Source: CAD feature listing. Evaluate the final solid. Frame: model axes, mm. Coordinates: 2 decimals unless noted, no trailing zeros. Loops run counter-clockwise (first coordinate to the right, second up) from the corner with the lowest first, then second, coordinate; pieces in that order, holes last. Notation, with made-up numbers: (-32.5, 33) - (18.5, 33) arc R27 cw to (18.5, 57) - close; hole circle Ø1 at (31.25, 40.5). An arc over 180 degrees is marked (long way). Use CSV: the item, a comma, the result in double quotes. Start each with the question number.
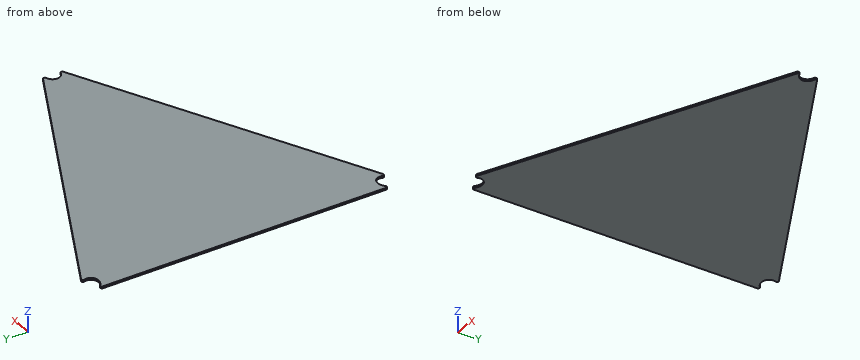
```python
from build123d import *

# Parameters (mm, degrees)
BOSS_EXTRUDE1_DEPTH = 3.175
FILLET1_START       = -1
FILLET1_DEPTH       = 5


with BuildPart() as part:
    # Sketch2 → Boss-Extrude1 (new body)
    with BuildSketch(Plane.XY):
        with BuildLine():
            Line((252.882647522, 18.233509916), (-227.808389099, 261.102259727))
            add(Edge.make_bspline(
                [(-227.808389099, 261.102259727), (-218.508408171, 256.403452033), (-217.090340448, 248.048262702), (-220.367085383, 242.285684549)],
                knots=[0.742781474, 0.742781474, 0.742781474, 0.742781474, 1, 1, 1, 1], degree=3, weights=[0.500416857, 0.490514251, 0.657041966, 1]))
            add(Edge.make_bspline(
                [(-220.367085383, 242.285684549), (-227.805809429, 229.203729887), (-247.735230176, 231.479633917), (-247.728634027, 251.479512649)],
                knots=[0, 0, 0, 0, 0.406744285, 0.406744285, 0.406744285, 0.406744285], degree=3, weights=[1, 0.457674286, 0.356524342, 0.696550168]))
            Line((-247.728634027, 251.479512649), (-247.88971408, -236.923885776))
            add(Edge.make_bspline(
                [(-247.88971408, -236.923885776), (-247.883118871, -216.926855588), (-227.957336221, -214.663599199), (-220.525871765, -227.745847533)],
                knots=[0.593296933, 0.593296933, 0.593296933, 0.593296933, 1, 1, 1, 1], degree=3, weights=[0.696446809, 0.356544847, 0.457729245, 1]))
            add(Edge.make_bspline(
                [(-220.525871765, -227.745847533), (-217.251599097, -233.509832332), (-218.672940969, -241.864237022), (-227.974334939, -246.55870873)],
                knots=[0, 0, 0, 0, 0.25721856, 0.25721856, 0.25721856, 0.25721856], degree=3, weights=[1, 0.65704192, 0.490514207, 0.500416861]))
            Line((-227.974334939, -246.55870873), (252.876255857, -3.870408269))
            add(Edge.make_bspline(
                [(252.876255857, -3.870408269), (240.565044662, -10.083953555), (231.629829811, -2.056184754), (231.628366282, 7.18068181)],
                knots=[0.684200569, 0.684200569, 0.684200569, 0.684200569, 1, 1, 1, 1], degree=3, weights=[0.534636521, 0.423812933, 0.578934092, 1]))
            add(Edge.make_bspline(
                [(231.628366282, 7.18068181), (231.626901898, 16.422942754), (240.567824747, 24.455563967), (252.882647522, 18.233509916)],
                knots=[0, 0, 0, 0, 0.315906176, 0.315906176, 0.315906176, 0.315906176], degree=3, weights=[1, 0.578791765, 0.423708096, 0.534748993]))
        make_face()
    extrude(amount=BOSS_EXTRUDE1_DEPTH)

    # Fillet1: read off the stored shape, not the designer's step
    # Fillet1 outline → Fillet1 (cut)
    with BuildSketch(Plane.XY.offset(FILLET1_START)):
        with BuildLine():
            Line((-247.728634027, 251.479512649), (-247.73250842, 239.732143832))
            ThreePointArc((-247.73250842, 239.732143832), (-246.154410329, 242.082124056), (-243.381643145, 241.512419941))
            add(Edge.make_bspline(
                [(-243.381643145, 241.512419941), (-246.348546976, 244.528882707), (-247.729754583, 248.081924898), (-247.728634027, 251.479512649)],
                knots=[1.290568731, 1.290568731, 1.290568731, 1.290568731, 1.406744285, 1.406744285, 1.406744285, 1.406744285], degree=3, weights=[0.513166576, 0.538303082, 0.599430946, 0.696550168]))
        make_face()
        with BuildLine():
            ThreePointArc((-243.536134042, -226.959195307), (-246.309281681, -227.52709022), (-247.885839538, -225.176065383))
            Line((-247.885839538, -225.176065383), (-247.88971408, -236.923885776))
            add(Edge.make_bspline(
                [(-247.88971408, -236.923885776), (-247.888593429, -233.526010078), (-246.504981138, -229.973706223), (-243.536134042, -226.959195307)],
                knots=[0.593296933, 0.593296933, 0.593296933, 0.593296933, 0.709466339, 0.709466339, 0.709466339, 0.709466339], degree=3, weights=[0.696446809, 0.599358264, 0.538257269, 0.513143822]))
        make_face()
        with BuildLine():
            add(Edge.make_bspline(
                [(-227.808389099, 261.102259727), (-223.785212041, 259.069552836), (-220.970894654, 255.819508956), (-219.668408897, 252.094046153)],
                knots=[0.742781474, 0.742781474, 0.742781474, 0.742781474, 0.855317926, 0.855317926, 0.855317926, 0.855317926], degree=3, weights=[0.500416857, 0.496084338, 0.525523694, 0.588734925]))
            ThreePointArc((-219.668408897, 252.094046153), (-218.944883502, 254.842497831), (-216.125289867, 255.199383475))
            Line((-216.125289867, 255.199383475), (-227.808389099, 261.102259727))
        make_face()
        with BuildLine():
            ThreePointArc((-216.289382855, -240.661240335), (-219.108792384, -240.303160787), (-219.831184056, -237.554444482))
            add(Edge.make_bspline(
                [(-219.831184056, -237.554444482), (-221.135109685, -241.279221567), (-223.950577298, -244.527893084), (-227.974334939, -246.55870873)],
                knots=[1.144682938, 1.144682938, 1.144682938, 1.144682938, 1.25721856, 1.25721856, 1.25721856, 1.25721856], degree=3, weights=[0.588733468, 0.525523222, 0.496084353, 0.500416861]))
            Line((-227.974334939, -246.55870873), (-216.289382855, -240.661240335))
        make_face()
        with BuildLine():
            Line((252.882647522, 18.233509916), (241.670605569, 23.898384866))
            ThreePointArc((241.670605569, 23.898384866), (243.055767599, 21.412939134), (241.265285671, 19.201539396))
            add(Edge.make_bspline(
                [(241.265285671, 19.201539396), (245.20247003, 20.400808532), (249.313639066, 20.036748495), (252.882647522, 18.233509916)],
                knots=[1.208515124, 1.208515124, 1.208515124, 1.208515124, 1.315906176, 1.315906176, 1.315906176, 1.315906176], degree=3, weights=[0.513767959, 0.490007402, 0.49700108, 0.534748993]))
        make_face()
        with BuildLine():
            ThreePointArc((241.25790796, -4.833713175), (243.047416072, -7.045891114), (241.661178159, -9.530728124))
            Line((241.661178159, -9.530728124), (252.876255857, -3.870408269))
            add(Edge.make_bspline(
                [(252.876255857, -3.870408269), (249.305839521, -5.672419724), (245.194273266, -6.034625453), (241.25790796, -4.833713175)],
                knots=[0.684200569, 0.684200569, 0.684200569, 0.684200569, 0.791591528, 0.791591528, 0.791591528, 0.791591528], degree=3, weights=[0.534636521, 0.49694978, 0.49001722, 0.513838842]))
        make_face()
    extrude(amount=FILLET1_DEPTH, mode=Mode.SUBTRACT)


solid = part.part
```
(1) Section A-A on y = 115.5. Output: boundary loops of the cut face in (x, z) (3 decimals), plus the area to 3 significant figures.
(2) Section B-B on x = -189.5. Output: boundary loops of the cut face in (y, z) (3 decimals), plus the area to 3 significant figures.
(3) Ray query, line 1 (Y direction, x = -84.5, z = 0.2); line 2 (X direction, y = 49.5, z = 2.8); line 3 (Y direction, x = 35, z = 0.85). Return the intervals inside material, ascending. Write a range as [from, to].
(4) Pin query (flat end, axial travel): pin 1 Ø1.5 at (x, z) = (160.5, 3) entering from +Y; pin 2 Ø1.5 at (y, z) = (174, 2.5) entering from -X. Return the tip coordinate at first contact, or that it passes through.
Solution:
1,outline,"(-247.773, 0) - (60.371, 0) - (60.371, 3.175) - (-247.773, 3.175) - close"
1,area,"978 mm²"
2,outline,"(-227.14, 0) - (241.747, 0) - (241.747, 3.175) - (-227.14, 3.175) - close"
2,area,"1,490 mm²"
3,line 1,"y = [-174.15, 188.7]"
3,line 2,"x = [-247.8, 191]"
3,line 3,"y = [-113.83, 128.32]"
4,pin 1,"stops at y = 65.29"
4,pin 2,"stops at x = -247.75"
